For this review, use the dimensioned drawing (mm, ordinates from the lowest corner) and the shaded views. Coordinates: 2 decimals unless noted, no trailing zeros. Write each loop counter-clockwise with the first axis right and the second up, starting at its lowest first coordinate (ties: lowest second). Pieces come first, ordered by that corner, then holes. Notation, with made-up numbers: M 23,-4 L 40,-4 A21 cw 40,12 Z; hole C 67,-20 d6. An arc over 180 degrees is marked long. Return JSON: item names as keys, results as strings. Group by question number.
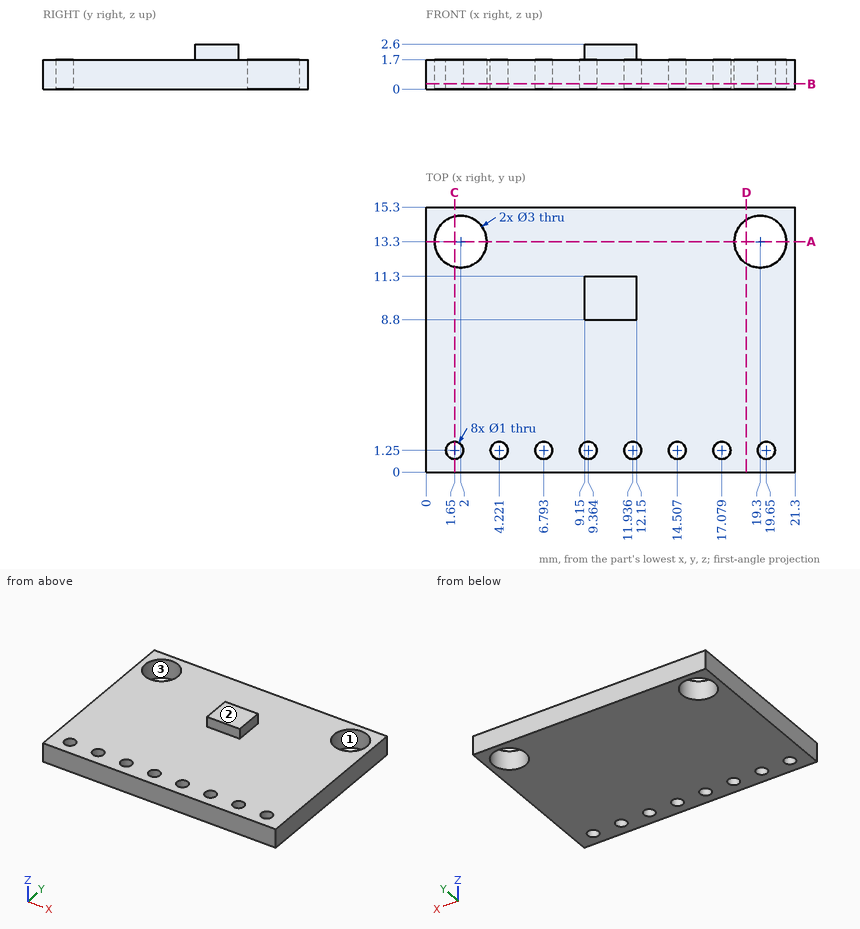
Item 1: For line 1 (Y direction, x = 2, z = 0.5) (1 decimal); line 2 (X direction, y = 14, z = 0.4) (1 decimal); line 3 (Y direction, x = 1.25, z = 0.7), list the stretches that pass through material, from the lowest coordinate up.
Item 2: Add section C-C (x = 1.65). Write out the cut boundary in (y, z).
Item 3: Add section A-A (y = 13.3). Write out the cut boundary in (x, z).
Item 4: For pin 1 (1.8 mm diameter, centred on x = 19.3, y = 13.3, fed in from +Z); pin 2 (5 mm diameter, centred on x = 12, y = 3, fed in from +Z), all flat-tipped, find the tip position at first contact; note any pin that passes through.
Item 5: Add section B-B (z = 0.3). Count the separate pieces of the cut face and the enclosed holes in it.
Item 6: Add section D-D (x = 18.5). Write out the cut boundary in (y, z).
Item 7: The part is to be moulded in two halves that separate along X. For the marked faces 1, 2 and 3, say which applies: pulls with the +X half, pulls with the -X half, needs draft (parallel to the pull), parting line crosses it, or undercut.
Geometry check:
{
 "1": {"line 1": "0 to 0.9, 1.6 to 11.8, 14.8 to 15.3", "line 2": "0 to 0.7, 3.3 to 18, 20.6 to 21.3", "line 3": "0 to 0.95, 1.55 to 12, 14.6 to 15.3"},
 "2": {"outline": "M 0,0 L 0.75,0 L 0.75,1.7 L 0,1.7 Z; M 1.75,0 L 11.84,0 L 11.84,1.7 L 1.75,1.7 Z; M 14.76,0 L 15.3,0 L 15.3,1.7 L 14.76,1.7 Z"},
 "3": {"outline": "M 0,0 L 0.5,0 L 0.5,1.7 L 0,1.7 Z; M 3.5,0 L 17.8,0 L 17.8,1.7 L 3.5,1.7 Z; M 20.8,0 L 21.3,0 L 21.3,1.7 L 20.8,1.7 Z"},
 "4": {"pin 1": "through", "pin 2": "z = 1.7"},
 "5": {"separate pieces": "1", "enclosed holes": "10"},
 "6": {"outline": "M 0,0 L 12.03,0 L 12.03,1.7 L 0,1.7 Z; M 14.57,0 L 15.3,0 L 15.3,1.7 L 14.57,1.7 Z"},
 "7": {"face 1": "undercut", "face 2": "needs draft", "face 3": "undercut"}
}
